```python
from build123d import *

# Parameters (mm, degrees)
SKETCH_1_W      = 68
SKETCH_1_H      = 44
SKETCH_1_R      = 1.5
EXTRUDE_1_DEPTH = 12
FILLET_1_SIZE   = 3


with BuildPart() as part:
    # 草图1 → 凸台-拉伸1 (new body)
    with BuildSketch(Plane(origin=(0, 0, 0), x_dir=(1, 0, 0), z_dir=(0, 1, 0))):
        with Locations((2.141772152, 0)):
            Rectangle(SKETCH_1_W, SKETCH_1_H)
        with Locations(Location((-28.358227848, -18.5, 0), (0, 0, 270))):
            Circle(SKETCH_1_R, mode=Mode.SUBTRACT)
        with Locations(Location((32.641772152, -18.5, 0), (0, 0, 90))):
            Circle(SKETCH_1_R, mode=Mode.SUBTRACT)
        with Locations(Location((32.641772152, 18.5, 0), (0, 0, 270))):
            Circle(SKETCH_1_R, mode=Mode.SUBTRACT)
        with Locations(Location((-28.358227848, 18.5, 0), (0, 0, 90))):
            Circle(SKETCH_1_R, mode=Mode.SUBTRACT)
    extrude(amount=EXTRUDE_1_DEPTH)

    # 圆角1
    # a fillet whose section is not a circle: 3 mm, written as the material it takes off along each edge
    with BuildSketch(Plane(origin=(-31.858227848, -7.5, -22), x_dir=(1, 0, 0), z_dir=(0, 1, 0))) as fillet_1_piece_1:
        with BuildLine():
            add(Edge.make_bspline([(FILLET_1_SIZE, 0), (FILLET_1_SIZE * 0.831801948466, 0), (FILLET_1_SIZE * 0.663603896932, 0), (FILLET_1_SIZE * 0.292893218813, -FILLET_1_SIZE * 0.0716919198361), (FILLET_1_SIZE * 0.0716919198361, -FILLET_1_SIZE * 0.292893218813), (0, -FILLET_1_SIZE * 0.663603896932), (0, -FILLET_1_SIZE * 0.831801948466), (0, -FILLET_1_SIZE)], knots=[0, 0, 0, 0, 0, 0, 0.5, 0.5, 1, 1, 1, 1, 1, 1], degree=5))
            Line((0, -FILLET_1_SIZE), (0, 0))
            Line((0, 0), (FILLET_1_SIZE, 0))
        make_face()
    extrude(amount=27, mode=Mode.SUBTRACT)
    with BuildSketch(Plane(origin=(36.141772152, -7.5, -22), x_dir=(-1, 0, 0), z_dir=(0, 1, 0)), Plane(origin=(-31.858227848, -7.5, 22), x_dir=(1, 0, 0), z_dir=(0, 1, 0)), Plane(origin=(36.141772152, -7.5, 22), x_dir=(0, 0, -1), z_dir=(0, 1, 0))) as fillet_1_piece_2:
        with BuildLine():
            add(Edge.make_bspline([(FILLET_1_SIZE, 0), (FILLET_1_SIZE * 0.831801948466, 0), (FILLET_1_SIZE * 0.663603896932, 0), (FILLET_1_SIZE * 0.292893218813, FILLET_1_SIZE * 0.0716919198361), (FILLET_1_SIZE * 0.0716919198361, FILLET_1_SIZE * 0.292893218813), (0, FILLET_1_SIZE * 0.663603896932), (0, FILLET_1_SIZE * 0.831801948466), (0, FILLET_1_SIZE)], knots=[0, 0, 0, 0, 0, 0, 0.5, 0.5, 1, 1, 1, 1, 1, 1], degree=5))
            Line((0, FILLET_1_SIZE), (0, 0))
            Line((0, 0), (FILLET_1_SIZE, 0))
        make_face()
    extrude(amount=27, mode=Mode.SUBTRACT)


solid = part.part
```
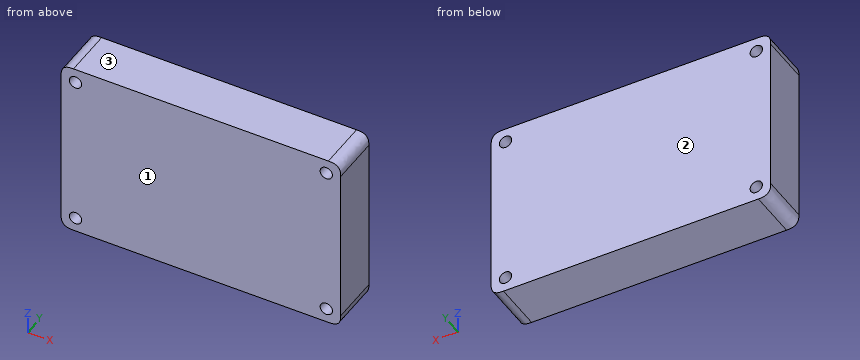
Check sheet for the modelled part. Datum: model origin and axes. Units: mm. Face numbers are marked on the shaded views. Round coordinates to 2 decimals unless told otherwise and drop trailing zeros. Write item = value, one per line. Start each with the question number.
Q1. Depth check by flat-ended pin: P1, Ø1.8, axis at x = -28.36, z = 18.5, coming from the -Y side. Enter the tip coordinate at first touch or a pass-through.
Q2. Release check for a two-part mould opening along Y. For the marked faces 1, 2 and 3 record: pulls with the +Y half, pulls with the -Y half, needs draft (parallel to the pull), parting line crosses it, or undercut.
Q3. Thickness scan on L1, parallel to X at y = 5, z = 18.5; L2, parallel to Z at x = 32.5, y = 2.5; L3, parallel to Z at x = -27, y = 9. Record the ranges inside material, lowest first.
Derived:
q1.P1 = through
q2.face_1 = pulls with the -Y half
q2.face_2 = pulls with the +Y half
q2.face_3 = needs draft
q3.L1 = -31.86 to -29.86, -26.86 to 31.14, 34.14 to 36.14
q3.L2 = -22 to -19.99, -17.01 to 17.01, 19.99 to 22
q3.L3 = -22 to -19.14, -17.86 to 17.86, 19.14 to 22
